Check sheet for the drawn part. Datum: minimum x, y, z corner. Units: mm. A direction names the side the tool comes from. Give positions to 0.01 mm unless a question says otherwise; leave off trailing zeros. Loops run counter-clockwise (first coordinate to the right, second up) from the corner with the lowest first, then second, coordinate; pieces in that order, holes last. Notation, with made-up numbers: (-7, -32.5) - (1, -32.5) arc R27 ccw to (1, -16.5) - close; hole circle Ø1 at (40.25, 10). An arc over 180 degrees is marked (long way). Use one line per item in the form item = value.
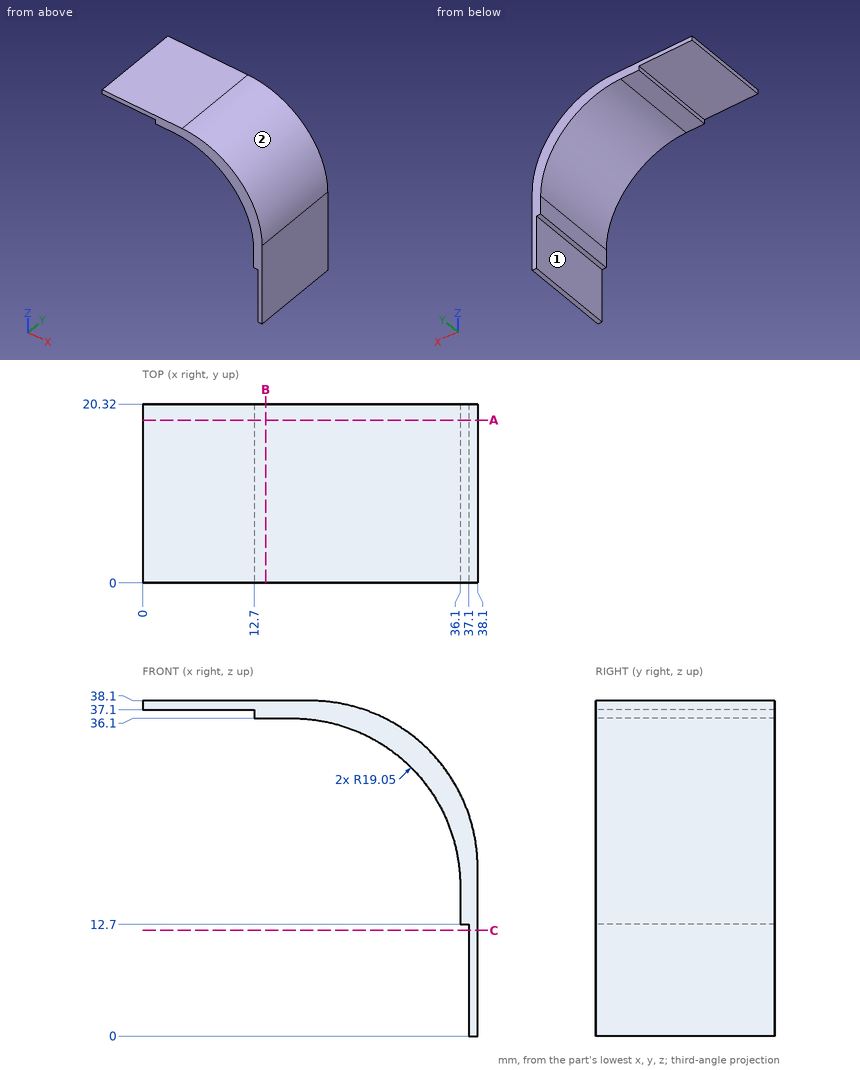
1. Section check C-C, the plane z = 12. Record the cut outline in (x, y).
Result set:
outline = (37.1, 0) - (38.1, 0) - (38.1, 20.32) - (37.1, 20.32) - close
2. Depth check by flat-ended pin: pin 1 Ø1.5 at (y, z) = (12.5, 23) entering from +X; pin 2 Ø10 at (x, y) = (27, 16) entering from -Z; pin 3 Ø5 at (y, z) = (11.5, 16) entering from -X. Enter the tip coordinate at first touch or a pass-through.
Result set:
pin_1 = 37.83
pin_2 = 28.86
pin_3 = 36.04
3. Tool access check on the marked faces 1 and 2. Record the directions out of +Z, -Z, +X, -X, +Y, -Y that give a thin tool (end or side, any length) a straight path to the whole face; none if there is none.
Result set:
face_1 = -Z, -X, +Y, -Y
face_2 = +Z, +X, +Y, -Y
4. Section check B-B, the plane x = 14. Record the cut outline in (y, z).
Result set:
outline = (0, 36.1) - (20.32, 36.1) - (20.32, 38.1) - (0, 38.1) - close
5. Section check A-A, the plane y = 18.5. Record the cut outline in (x, z).
Result set:
outline = (0, 37.1) - (12.7, 37.1) - (12.7, 36.1) - (17.05, 36.1) arc R19.05 cw to (36.1, 17.05) - (36.1, 12.7) - (37.1, 12.7) - (37.1, 0) - (38.1, 0) - (38.1, 19.05) arc R19.05 ccw to (19.05, 38.1) - (0, 38.1) - close
6. Scan lines: probe 1 along X at (y, z) = (7.5, 14); probe 2 along Z at (x, y) = (7.5, 7.75). Record each from-to range of solid material in increasing order.
Result set:
probe_1 = 36.1 to 38.1
probe_2 = 37.1 to 38.1
